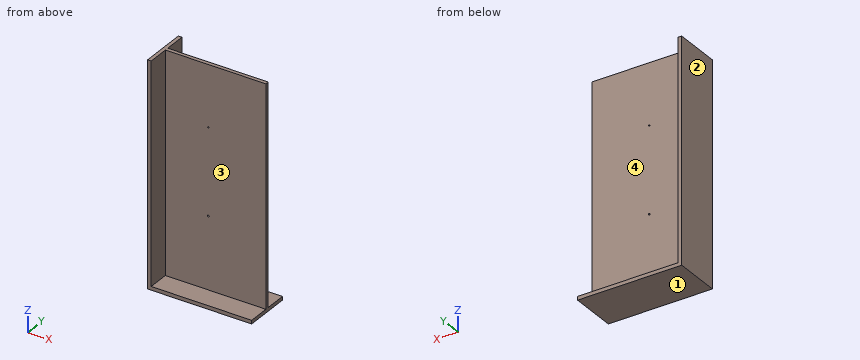
from build123d import *

# Parameters (mm, degrees)
F1_DEPTH = 193.675
F2_W     = 92.075
F2_H     = 41.275
F3_DEPTH = 3.175
F4_R     = 0.79375
F4_R_2   = 0.620834
F5_DEPTH = 3.175


with BuildPart() as f1:
    # F0 (on Top) → F1 (new body)
    with BuildSketch(Plane.XY):
        Polygon((0, 1.5875), (0, 20.6375), (-3.175, 20.6375), (-3.175, -20.6375), (0, -20.6375), (0, -1.5875), (88.9, -1.5875), (88.9, 1.5875), align=None)
    extrude(amount=F1_DEPTH)

    # F2 (on face) → F3 (join)
    with BuildSketch(Plane(origin=(0, 0, 0), x_dir=(1, 0, 0), z_dir=(0, 0, -1))):
        with Locations((42.8625, 0)):
            Rectangle(F2_W, F2_H)
    extrude(amount=F3_DEPTH)

    # F4 (on face) → F5 (cut, through all)
    with BuildSketch(Plane.XZ.offset(1.5875)):
        with Locations((38.1, 63.5)):
            Circle(F4_R)
        with Locations((38.1, 139.7)):
            Circle(F4_R_2)
    extrude(amount=-F5_DEPTH, mode=Mode.SUBTRACT)


solid = f1.part
Work out the finished part from the listing and answer in its coordinate system (mm). Face numbers are marked on the shaded views. A direction names the side the tool comes from. Round coordinates to 2 decimals unless told otherwise and drop trailing zeros. Loops run counter-clockwise (first coordinate to the right, second up) from the corner with the lowest first, then second, coordinate; pieces in that order, holes last. Notation, with made-up numbers: M 83,21 L 115,21 A27 cw 115,48 Z; hole C 1,78.5 d10. An arc over 180 degrees is marked long. One line per question, with ' | ' between items. Start each with the question number.
(1) A cutting plane is placed at A-A on z = 17.5. Write down the section's boundary in (x, y) (1 decimal), plus the area to 3 significant figures.
(2) Find the intervals of material crossed by line 1 (Z direction, x = 38.1, y = -0.55) (3 decimals); line 2 (X direction, y = -0.1, z = 63.5) (3 decimals); line 3 (X direction, y = 0.05, z = 139.7) (3 decimals), in increasing order.
(3) A cutting plane is placed at C-C on x = 34.5. Write down the section's boundary in (y, z) (1 decimal), plus the area to 3 significant figures.
(4) For a pull along Z with two mould halves and no side action, classify the marked faces 1 and 2 as released by +Z, released by -Z, zero draft, split by the parting line, or undercut.
(5) A cutting plane is placed at B-B on y = 13. Write down the section's boundary in (x, z) (3 decimals).
(6) A tool of negligible diameter and unlimited length cuts with its end or side. For the marked faces 3 and 4, from which of +Z, -Z, +X, -X, +Y, -Y can it reach the whole face along a straight path? Write none if from no direction.
(7) Flat-ended cylindrical pins translate along their axes: pin 1 Ø5.5 at (x, y) = (22.5, -10.5) entering from +Z; pin 2 Ø10 at (x, z) = (36.5, 83.5) entering from +Y; pin 3 Ø4 at (y, z) = (12, 97) entering from +X; pin 4 Ø1.3 at (x, z) = (38.1, 63.5) entering from +Y. Find the tip coordinate at first contact, or state that the pin passes through.
Geometry check:
1) outline: M -3.2,-20.6 L 0,-20.6 L 0,-1.6 L 88.9,-1.6 L 88.9,1.6 L 0,1.6 L 0,20.6 L -3.2,20.6 Z | area: 413 mm²
2) line 1: z = -3.175 to 62.706, 64.294 to 139.079, 140.321 to 193.675 | line 2: x = -3.175 to 37.306, 38.894 to 88.9 | line 3: x = -3.175 to 37.479, 38.721 to 88.9
3) outline: M -20.6,-3.2 L 20.6,-3.2 L 20.6,0 L 1.6,0 L 1.6,193.7 L -1.6,193.7 L -1.6,0 L -20.6,0 Z | area: 746 mm²
4) face 1: released by -Z | face 2: zero draft
5) outline: M -3.175,-3.175 L 88.9,-3.175 L 88.9,0 L 0,0 L 0,193.675 L -3.175,193.675 Z
6) face 3: +Z, +X, -Y | face 4: +Z, +X, +Y
7) pin 1: stops at z = 0 | pin 2: stops at y = 1.59 | pin 3: stops at x = 0 | pin 4: passes through
